Source: CAD feature listing. Evaluate the final solid. Frame: model axes, mm. Face numbers are marked on the shaded views. A direction names the side the tool comes from. Give positions to 0.01 mm unless a question says otherwise; leave off trailing zeros. Write each loop counter-clockwise with the first axis right and the second up, starting at its lowest first coordinate (ties: lowest second). Pieces come first, ordered by that corner, then holes. Notation, with made-up numbers: (-18, 49.25) - (-14, 49.25) arc R29 ccw to (-14, 81.25) - close; hole circle Ø6 at (-37.75, 25). An arc over 180 degrees is marked (long way). One line per question, with ' | ' between items. Start each with the question number.
(1) Ray query, line 1 (X direction, y = -60, z = 0.75); line 2 (Y direction, x = 15.5, z = -1.75); line 3 (Y direction, x = 4, z = -5.5). Return the intervals inside material, ascending. Write a range as [from, to].
(2) Section A-A, the plane x = 0. Return loops of the section in (y, z) (1 decimal), plus the area to 3 significant figures.
(3) Section D-D, the plane x = 5. Return loops of the section in (y, z).
(4) Section B-B, the plane x = -10. Return loops of the section in (y, z).
(5) Section C-C, the plane z = 1.25. State how many separate pieces and enclosed holes the cut face has, plus the area to 3 significant figures.
(6) Access query for the marked faces 1, 2 and 3. Directions: +Z, -Z, +X, -X, +Y, -Y. A direction counts if a zero-diameter tool reaches every point of the face in a straight line with its end or side. Return the directions, or none.
(7) Pin query (flat end, axial travel): pin 1 (22 mm diameter, centred on x = 7, y = -80, fed in from -Z); pin 2 (3.5 mm diameter, centred on x = 5.5, z = -3.5, fed in from -Y); pin 3 (5 mm diameter, centred on y = -31.5, z = -4, fed in from -X). Return the tip coordinate at first contact, or that it passes through.
Autodesk Inventor part; units mm, degrees
ref_plane "YZ Plane" through (0, 0, 0) normal (1, 0, 0) x (0, 1, 0)
ref_plane "XZ Plane" through (0, 0, 0) normal (0, 1, 0) x (-1, 0, 0)
sketch "Sketch1" plane through (0, 0, 0) normal (0, 0, 1) x (1, 0, 0)
  line L0 (0, 128.9005) -> (0, -151.1555)
  line L1 (-57.1993, 0) -> (35.1957, 0)
  line L2 (21.9964, -103.8925) -> (-21.9964, -103.8925)
  line L3 (-21.9964, -103.8925) -> (-21.9964, -18.4723)
  line L4 (-21.9964, -18.4723) -> (21.9964, -18.4723)
  line L5 (21.9964, -18.4723) -> (21.9964, -103.8925)
  line L6 (21.9964, -103.8925) -> (-21.9964, -18.4723) construction
  line L7 (-21.9964, -103.8925) -> (21.9964, -18.4723) construction
  line L8 (15.5, -90.8175) -> (-15.5, -90.8175) construction
  line L9 (-15.5, -90.8175) -> (-15.5, -59.8175) construction
  line L10 (-15.5, -59.8175) -> (15.5, -59.8175) construction
  line L11 (15.5, -59.8175) -> (15.5, -90.8175) construction
  line L12 (15.5, -90.8175) -> (-15.5, -59.8175) construction
  line L13 (-15.5, -90.8175) -> (15.5, -59.8175) construction
  line L14 (0, -111.1475) -> (0, -39.4875) construction
  line L15 (-15.5, -64.8975) -> (-15.5, -54.7375) construction
  line L16 (-13.849, -64.8975) -> (-13.849, -54.7375)
  line L17 (-17.151, -54.7375) -> (-17.151, -64.8975)
  arc A0 (-17.151, -64.8975) -> (-13.849, -64.8975) centre (-15.5, -64.8975) ccw
  arc A1 (-13.849, -54.7375) -> (-17.151, -54.7375) centre (-15.5, -54.7375) ccw
  arc A2 (17.151, -54.7375) -> (13.849, -54.7375) centre (15.5, -54.7375) ccw
  line L18 (17.151, -64.8975) -> (17.151, -54.7375)
  line L19 (15.5, -64.8975) -> (15.5, -54.7375) construction
  line L20 (13.849, -54.7375) -> (13.849, -64.8975)
  arc A3 (13.849, -64.8975) -> (17.151, -64.8975) centre (15.5, -64.8975) ccw
  arc A4 (-13.849, -85.7375) -> (-17.151, -85.7375) centre (-15.5, -85.7375) ccw
  line L21 (-13.849, -95.8975) -> (-13.849, -85.7375)
  line L22 (-15.5, -95.8975) -> (-15.5, -85.7375) construction
  line L23 (-17.151, -85.7375) -> (-17.151, -95.8975)
  arc A5 (-17.151, -95.8975) -> (-13.849, -95.8975) centre (-15.5, -95.8975) ccw
  arc A6 (17.151, -85.7375) -> (13.849, -85.7375) centre (15.5, -85.7375) ccw
  line L24 (17.151, -95.8975) -> (17.151, -85.7375)
  line L25 (15.5, -95.8975) -> (15.5, -85.7375) construction
  line L26 (13.849, -85.7375) -> (13.849, -95.8975)
  arc A7 (13.849, -95.8975) -> (17.151, -95.8975) centre (15.5, -95.8975) ccw
  line L27 (0, -70.2375) -> (0, -80.3975) construction
  line L28 (13.0175, -70.2375) -> (13.0175, -80.3975)
  line L29 (-13.0175, -80.3975) -> (-13.0175, -70.2375)
  arc A8 (13.0175, -70.2375) -> (-13.0175, -70.2375) centre (0, -70.2375) ccw
  arc A9 (-13.0175, -80.3975) -> (13.0175, -80.3975) centre (0, -80.3975) ccw
  point P0 (0, -75.3175)
  point P1 (-44, 88.8925)
  point P2 (15.5, -59.8175)
  point P3 (-15.5, -90.8175)
  point P4 (15.5, -90.8175)
  point P5 (0, -75.3175)
  dimension "d5" = 31
  dimension "d6" = 31
  dimension "d10" = 28.575
  dimension "d11" = 3.302
  dimension "d12" = 10.16
  dimension "d15" = 31
  dimension "d18" = 31
  dimension "d45" = 5.08
  dimension "d51" = 43.9928
  dimension "d62" = 5.08
  dimension "d63" = 85.4202
  dimension "d77" = 21.9964
extrude "Extrusion1" add sketch "Sketch1" along normal blind 3.302
extrude "Extrusion3" cut sketch "Sketch1" along normal through all contours A8 L28 A9 L0 | L0 A9 L29 A8
sketch "Sketch3" plane through (0, 0, 3.302) normal (0, 0, 1) x (1, 0, 0)
  point P0 (0, 0)
  point P1 (-44, 68.8925)
  point P2 (44, 88.8925)
  point P3 (44, 68.8925)
  point P4 (-44, 88.8925)
hole "Hole2" at (-44, 68.8925, 3.302) at (44, 88.8925, 3.302) at (44, 68.8925, 3.302) at (-44, 88.8925, 3.302) direction (0, 0, -1) diameter 7.0104 end through all
sketch "Sketch5" plane through (0, 0, 0) normal (1, 0, 0) x (0, 1, 0)
  line L0 (-18.4723, 0) -> (-103.8925, 0)
  line L1 (-18.4723, 0) -> (-18.4723, 3.302)
  line L2 (-103.8925, 3.302) -> (-18.4723, 3.302)
  line L3 (-103.8925, 0) -> (-103.8925, 3.302)
  line L4 (-18.4723, 0) -> (-103.8925, 0)
  line L5 (-18.4723, 0) -> (-49.1047, 0)
  line L6 (-49.1047, 0) -> (-49.1047, -4.572)
  line L7 (-49.1047, -4.572) -> (-18.4723, -4.572)
  line L8 (-18.4723, -4.572) -> (-18.4723, 0)
  line L9 (-49.1047, -4.572) -> (-41.4847, -4.572)
  line L10 (-41.4847, -4.572) -> (-41.4847, -7.112)
  line L11 (-41.4847, -7.112) -> (-49.1047, -7.112)
  line L12 (-49.1047, -7.112) -> (-49.1047, -4.572)
  point P0 (0, 0)
  dimension "d70" = 23.0124
  dimension "d71" = 7.62
  dimension "d72" = 4.572
  dimension "d73" = 2.54
extrude "Extrusion4" add sketch "Sketch5" against normal blind 15.24 and the other way blind 21.9964 contours L8 L7 L6 L0 | L7 L10 L11 L12
fillet "Fillet2" radius 7.62 2 edges at (-21.9964, -103.8925, 1.651) (21.9964, -103.8925, 1.651)
sketch "Sketch6" plane through (0, 0, 3.302) normal (0, 0, 1) x (1, 0, 0)
  line L0 (-15.24, -41.4847) -> (21.9964, -41.4847)
  line L1 (21.9964, -96.2725) -> (21.9964, -18.4723)
  point P0 (0, 0)
  point P1 (11.9964, -25.4827)
  point P2 (-8.0036, -25.4827)
  dimension "d78" = 10
  dimension "d79" = 20
  dimension "d80" = 16.002
hole "Hole4" at (-8.0036, -25.4827, 3.302) at (11.9964, -25.4827, 3.302) direction (0, 0, -1) diameter 6.604 end through all
sketch "Sketch7" plane through (0, 0, 0) normal (0, 0, -1) x (-1, 0, 0)
  line L0 (15.24, -41.4847) -> (15.24, -49.1047)
  line L1 (15.24, -49.1047) -> (-21.9964, -49.1047)
  line L2 (21.9964, -18.4723) -> (15.24, -18.4723)
  line L3 (21.9964, -96.2725) -> (21.9964, -18.4723)
  line L4 (15.24, -49.1047) -> (21.9964, -49.1047)
  line L5 (21.9964, -49.1047) -> (21.9964, -18.4723)
  line L6 (21.9964, -18.4723) -> (15.24, -18.4723)
  line L7 (15.24, -18.4723) -> (15.24, -49.1047)
  point P0 (0, 0)
extrude "Extrusion5" cut sketch "Sketch7" against normal up to next
fillet "Fillet3" radius 3.175 2 edges at (-15.24, -49.1047, 1.651) (-21.9964, -49.1047, 1.651)
sketch "Sketch8" plane through (21.9964, -41.4847, -4.572) normal (0, 0, -1) x (-1, 0, 0)
  circle A0 centre (30, 16.002) radius 3.302
  circle A1 centre (10, 16.002) radius 3.302
  line L0 (37.2364, 0) -> (0, 0)
  line L1 (37.2364, 23.0124) -> (37.2364, 0)
  line L2 (37.2364, 23.0124) -> (0, 23.0124)
  line L3 (0, 0) -> (0, 23.0124)
  line L4 (0, 0) -> (8.89, 0)
  line L5 (8.89, 0) -> (8.89, 4.445)
  line L6 (8.89, 4.445) -> (0, 4.445)
  line L7 (0, 4.445) -> (0, 0)
  point P0 (21.9964, 41.4847)
  dimension "d91" = 4.445
  dimension "d92" = 8.89
extrude "Extrusion6" cut sketch "Sketch8" against normal up to surface (4.572 mm away) contours L0 L3 L6 L5
fillet "Fillet4" radius 2.032 2 edges at (13.1064, -41.4847, -2.286) (13.1064, -37.0397, -2.286)
equation "\"d15\" = d6"
equation "\"d18\" = d6"
equation "\"d77\" = 0.5 * d51"
equation "\"d74\" = 0.5 * d51"
properties part number "J008087" material "ALUMINUM, 6061-T651"
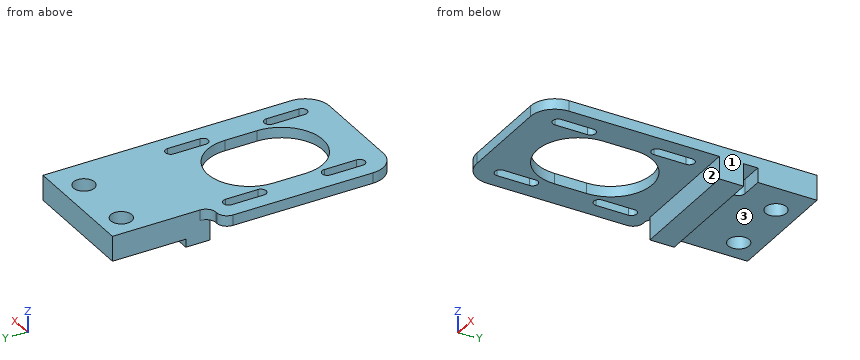
Check sheet entries:
1) line 1: [-22, -17.15], [-13.85, -8.04], [8.04, 13.85], [17.15, 22] | line 2: [-49.1, -41.48], [-37.04, -18.47] | line 3: [-49.1, -41.48]
2) outline: (-103.9, 0) - (-93.4, 0) - (-93.4, 3.3) - (-103.9, 3.3) - close; (-57.2, 0) - (-49.1, 0) - (-49.1, -7.1) - (-41.5, -7.1) - (-41.5, -4.6) - (-18.5, -4.6) - (-18.5, 3.3) - (-57.2, 3.3) - close | area: 322 mm²
3) outline: (-103.89, 0) - (-92.42, 0) - (-92.42, 3.3) - (-103.89, 3.3) - close; (-58.22, 0) - (-49.1, 0) - (-49.1, -7.11) - (-41.48, -7.11) - (-41.48, -4.57) - (-18.47, -4.57) - (-18.47, 3.3) - (-58.22, 3.3) - close
4) outline: (-103.89, 0) - (-88.73, 0) - (-88.73, 3.3) - (-103.89, 3.3) - close; (-61.9, 0) - (-49.1, 0) - (-49.1, -7.11) - (-41.48, -7.11) - (-41.48, -4.57) - (-28.11, -4.57) - (-28.11, 3.3) - (-61.9, 3.3) - close; (-22.85, -4.57) - (-18.47, -4.57) - (-18.47, 3.3) - (-22.85, 3.3) - close
5) separate pieces: 1 | enclosed holes: 7 | area: 2,490 mm²
6) face 1: +Z, -Z, +X, +Y, -Y | face 2: -Z, +X, -X, -Y | face 3: -Z, +X, -X, +Y
7) pin 1: z = 0 | pin 2: y = -49.1 | pin 3: x = -15.24
